Job drawing, mm, ordinate dimensions from the low corner. One solid piece. Round coordinates to 2 decimals unless told otherwise and drop trailing zeros. Loops run counter-clockwise (first coordinate to the right, second up) from the corner with the lowest first, then second, coordinate; pieces in that order, holes last.
1) Band-saw the part on B-B, the plane x = 67. Write the cut outline in (y, z), then the cut area to 4 significant figures.
2) Band-saw the part on C-C, the plane x = 221. Write the cut outline in (y, z), then the cut area to 3 significant figures.
3) Band-saw the part on A-A, the plane y = 0.95. State how many separate pieces and enclosed holes the cut face has, then the cut area to 3 significant figures.
4) Probe line 1 (Z direction, x = 109, y = 2.1); line 2 (Z direction, x = 47.5, y = 1.55); line 3 (X direction, y = 1.2, z = 23). List the from-to ranges inside material, lowest first.
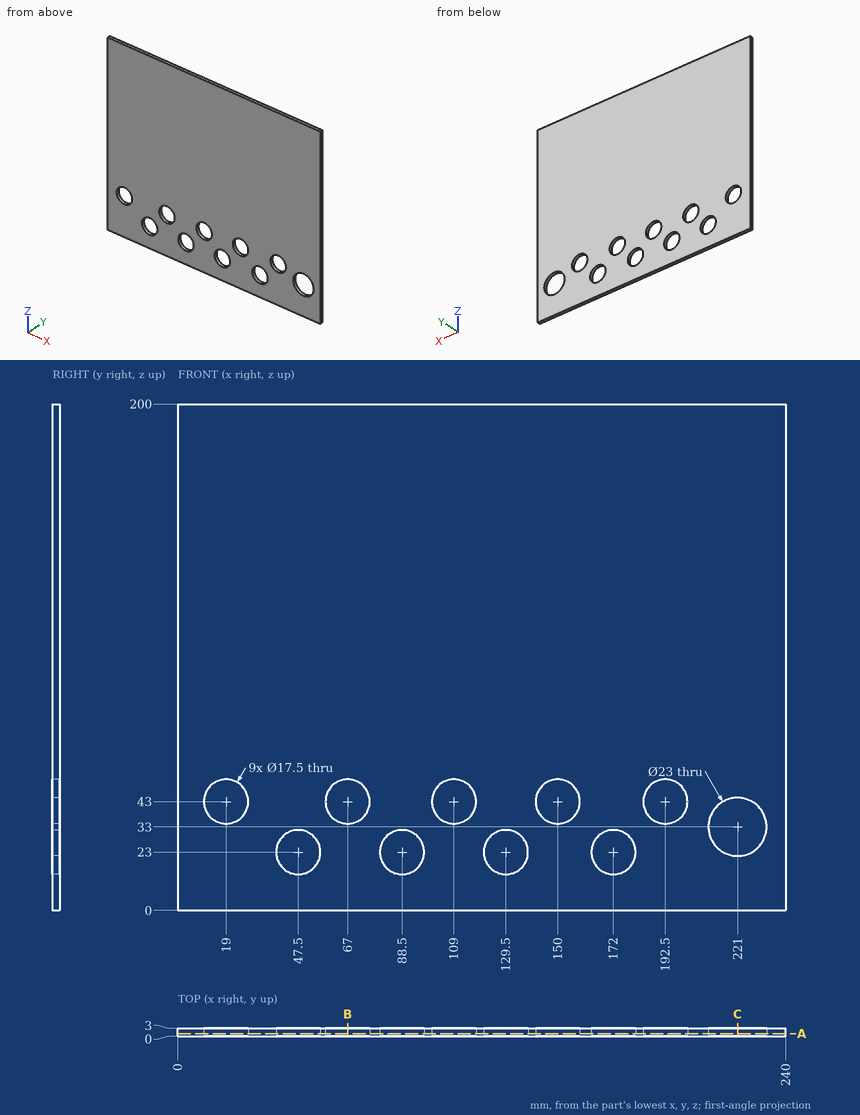
Reported:
1. outline: (0, 0) - (3, 0) - (3, 34.25) - (0, 34.25) - close; (0, 51.75) - (3, 51.75) - (3, 200) - (0, 200) - close
1. area: 547.5 mm2
2. outline: (0, 0) - (3, 0) - (3, 21.5) - (0, 21.5) - close; (0, 44.5) - (3, 44.5) - (3, 200) - (0, 200) - close
2. area: 531 mm2
3. separate pieces: 1
3. enclosed holes: 10
3. area: 45,400 mm2
4. line 1: z = 0 to 34.25, 51.75 to 200
4. line 2: z = 0 to 14.25, 31.75 to 200
4. line 3: x = 0 to 38.75, 56.25 to 79.75, 97.25 to 120.75, 138.25 to 163.25, 180.75 to 215.32, 226.68 to 240
